The listing builds one solid part. Answer for the finished solid, in the listing's coordinates (mm). A direction names the side the tool comes from. Round coordinates to 2 decimals unless told otherwise and drop trailing zeros. Write each loop counter-clockwise with the first axis right and the second up, starting at its lowest first coordinate (ties: lowest second). Pieces come first, ordered by that corner, then holes. Notation, with made-up numbers: (-16, 5.25) - (-5, 5.25) arc R16 ccw to (-5, 19.25) - close; hole circle Ø7 at (75.25, -4). An arc over 180 degrees is marked (long way). Return JSON: item names as keys, results as strings. Group by question number.
(1) Find the intervals of material crossed by line 1 along X through (y, z) = (-5.5, 2.45); line 2 along Y through (x, z) = (20.3, 1.65); line 3 along X through (y, z) = (-14.5, 1.7), in increasing order. Write a range as [from, to].
(2) Which of the six approach directions +Z, -Z, +X, -X, +Y, -Y give full straight-line access (tool end or side, diameter ignored) to faces 1 (the flat face through (19.593, -7, 1)), 2 (the flat face through (19, -8, 2.6))?
(3) Section A-A, the plane z = 0.7 is taken. Write down the section's boundary in (x, y).
(4) This flat-tipped pin is pushed along its axis until it touches: pin 1 (1.5 mm diameter, centred on x = 19.5, z = 2, fed in from -Y). Where does it stop, or does it pass through?
(5) Section B-B, the plane y = -3.5 is taken. Write down the section's boundary in (x, z), then the cut area to 3 significant figures.
(6) Section C-C, the plane x = 20 is taken. Write down the section's boundary in (y, z), then the cut area to 3 significant figures.
Autodesk Inventor part; units mm, degrees
ref_plane "YZ Plane" through (0, 0, 0) normal (1, 0, 0) x (0, 1, 0)
ref_plane "XZ Plane" through (0, 0, 0) normal (0, 1, 0) x (-1, 0, 0)
ref_plane "XY Plane" through (0, 0, 0) normal (0, 0, 1) x (1, 0, 0)
sketch "Sketch1" plane through (0, 0, 0) normal (0, 0, 1) x (1, 0, 0)
  line L0 (2, -10.465368) -> (4.697799, -10.465368) construction
  line L1 (0, 0) -> (50, 0)
  line L2 (50, 0) -> (50, -50)
  line L3 (50, -50) -> (0, -50)
  line L4 (0, -50) -> (0, 0)
  line L5 (2.4, -2.4) -> (47.6, -2.4)
  line L6 (47.6, -2.4) -> (47.6, -47.6)
  line L7 (47.6, -47.6) -> (2.4, -47.6)
  line L8 (2.4, -47.6) -> (2.4, -2.4)
  line L9 (2.4, -2.4) -> (47.6, -47.6) construction
  line L10 (47.6, -2.4) -> (2.4, -47.6) construction
  circle A0 centre (25, -25) radius 19.375
  circle A1 centre (25, -25) radius 14.5
  circle A2 centre (25, -25) radius 4.175
  circle A3 centre (31.679764, -18.320236) radius 2.65
  circle A4 centre (25, -15.553387) radius 2.65
  circle A5 centre (18.320236, -18.320236) radius 2.65
  circle A6 centre (15.553387, -25) radius 2.65
  circle A7 centre (18.320236, -31.679764) radius 2.65
  circle A8 centre (25, -34.446613) radius 2.65
  circle A9 centre (31.679764, -31.679764) radius 2.65
  circle A10 centre (34.446613, -25) radius 2.65
  line L11 (50, -25) -> (-10.932785, -25) construction
  line L12 (33.553597, -16.446403) -> (35.253048, -14.746952)
  line L13 (33.553597, -33.553597) -> (35.253048, -35.253048)
  arc A11 (16.446403, -16.446403) -> (16.447482, -33.554675) centre (24.992317, -25) ccw
  line L14 (16.446403, -16.446403) -> (14.746952, -14.746952)
  line L15 (16.447482, -33.554675) -> (14.746952, -35.253048)
  line L16 (3.4, -3.4) -> (46.6, -3.4)
  line L17 (46.6, -3.4) -> (46.6, -46.6)
  line L18 (46.6, -46.6) -> (3.4, -46.6)
  line L19 (3.4, -46.6) -> (3.4, -3.4)
  line L20 (46.6, -46.6) -> (43.6, -46.6)
  line L21 (43.6, -46.6) -> (43.6, -43.6)
  line L22 (43.6, -43.6) -> (46.6, -43.6)
  line L23 (46.6, -43.6) -> (46.6, -46.6)
  line L24 (43.6, -43.6) -> (38.700194, -43.6)
  line L25 (38.700194, -43.6) -> (38.700194, -38.700194)
  line L26 (38.700194, -38.700194) -> (43.6, -38.700194)
  line L27 (43.6, -38.700194) -> (43.6, -43.6)
  line L28 (43.6, -38.700194) -> (46.6, -38.700194)
  line L29 (46.6, -38.700194) -> (46.6, -35.700194)
  line L30 (46.6, -35.700194) -> (43.6, -35.700194)
  line L31 (43.6, -35.700194) -> (43.6, -38.700194)
  line L32 (46.6, -35.700194) -> (42.820879, -35.700194)
  line L33 (42.820879, -35.700194) -> (42.820879, -32.603085)
  line L34 (42.820879, -32.603085) -> (46.6, -32.603085)
  line L35 (46.6, -32.603085) -> (46.6, -35.700194)
  line L36 (38.700194, -43.6) -> (35.700194, -43.6)
  line L37 (35.700194, -43.6) -> (35.700194, -46.6)
  line L38 (35.700194, -46.6) -> (38.700194, -46.6)
  line L39 (38.700194, -46.6) -> (38.700194, -43.6)
  line L40 (35.700194, -46.6) -> (32.383701, -46.6)
  line L41 (32.383701, -46.6) -> (32.383701, -42.912889)
  line L42 (32.383701, -42.912889) -> (35.700194, -42.912889)
  line L43 (35.700194, -42.912889) -> (35.700194, -46.6)
  line L44 (23.5, -43.2) -> (26.5, -43.2)
  line L45 (26.5, -43.2) -> (26.5, -50)
  line L46 (26.5, -50) -> (23.5, -50)
  line L47 (23.5, -50) -> (23.5, -43.2)
  line L48 (23.5, -43.2) -> (26.5, -50) construction
  line L49 (26.5, -43.2) -> (23.5, -50) construction
  circle A12 centre (7.947368, -7.947368) radius 4.547368
  circle A13 centre (42.052632, -7.947368) radius 4.547368
  line L50 (2.4, -47.6) -> (2.4, -50)
  line L51 (47.6, -47.6) -> (47.6, -50)
  line L52 (22.407108, -14.233364) -> (20.194069, -16.446403)
  line L53 (25, 8.52179) -> (25, -70.2) construction
  line L54 (18.320236, -8.83287) -> (18.320236, -33.554675) construction
  line L55 (18.320236, -14.57257) -> (20.194069, -16.446403)
  line L56 (18.320236, -14.57257) -> (20.533275, -12.359531)
  line L57 (22.407108, -14.233364) -> (20.533275, -12.359531)
  line L58 (18.320236, -14.57257) -> (19.593028, -13.299778)
  line L59 (19.593028, -13.299778) -> (20.86582, -14.57257)
  line L60 (20.86582, -14.57257) -> (19.593028, -15.845362)
  line L61 (31.679764, -14.57257) -> (29.466725, -12.359531)
  line L62 (27.592892, -14.233364) -> (29.466725, -12.359531)
  line L63 (27.592892, -14.233364) -> (29.805931, -16.446403)
  line L64 (31.679764, -14.57257) -> (29.805931, -16.446403)
  line L65 (19.593028, 0) -> (17.593028, 0)
  line L66 (17.593028, 0) -> (17.593028, -16.836985)
  line L67 (17.593028, -16.836985) -> (19.593028, -16.836985)
  line L68 (19.593028, -16.836985) -> (19.593028, 0)
  line L69 (19.593028, -15.845362) -> (18.601406, -16.836985)
  point P0 (25, -46.6)
  point P1 (26.5, -44.316848)
  point P2 (26.5, -46.6)
  point P3 (42.052632, -3.4)
  point P4 (46.6, -7.947368)
  point P5 (3.4, -7.947368)
  point P6 (7.947368, -3.4)
  point P7 (26.5, -47.6)
  point P8 (23.5, -47.6)
  dimension "d12" = 5.3
  dimension "d5" = 50
  dimension "d6" = 50
  dimension "d7" = 45.2
  dimension "d8" = 45.2
  dimension "d9" = 38.75
  dimension "d10" = 29
  dimension "d11" = 8.35
  dimension "d13" = 360
  dimension "d14" = 2.4
  dimension "d15" = 2.4
  dimension "d16" = 1
  dimension "d17" = 1
  dimension "d18" = 1
  dimension "d19" = 3
  dimension "d20" = 3
  dimension "d21" = 3
  dimension "d22" = 3
  dimension "d23" = 3
  dimension "d24" = 3
  dimension "d25" = 3
  dimension "d26" = 1.8
  dimension "d27" = 2
extrude "Extrusion1" add sketch "Sketch1" along normal blind 2.6 contours L1 L68 L5 L66 | L5 L68 L16 L66 | L16 L68 A0 L66 | A0 L68 A1 L66 | A1 L68 L56 L55 L69 A5 L66 | A5 L69 L67 L66 | L68 L55 L56 | L59 L60 L68
properties part number "baseHook"
Working result:
{
 "1": {"line 1": "x = [17.59, 19.59]", "line 2": "y = [-15.14, -14.01]", "line 3": "x = [17.59, 20.79]"},
 "2": {"face 1": "+Z, -Z, +X, +Y", "face 2": "+Z, +X, -X, +Y, -Y"},
 "3": {"outline": "(17.59, -16.84) - (18.6, -16.84) - (19.59, -15.85) - (20.87, -14.57) - (19.59, -13.3) - (19.59, 0) - (17.59, 0) - close"},
 "4": {"pin 1": "stops at y = -16.69"},
 "5": {"outline": "(17.59, 0) - (19.59, 0) - (19.59, 2.6) - (17.59, 2.6) - close", "area": "5.20 mm^2"},
 "6": {"outline": "(-15.44, 0) - (-13.71, 0) - (-13.71, 2.6) - (-15.44, 2.6) - close", "area": "4.50 mm^2"}
}
